Check sheet for the modelled part. Datum: model origin and axes. Units: mm. A direction names the side the tool comes from. Give positions to 0.01 mm unless a question says otherwise; leave off trailing zeros. Order: outer loops, then holes, each group sorted by start corner. A loop starts at its lowest first (then second) coordinate and runs counter-clockwise, first axis right, second up.
Autodesk Inventor part; units mm, degrees
ref_plane "РабПлоскость1" through (-1, 17.5, -4.0985) normal (0, 0, -1) x (-1, 0, 0)
ref_plane "YZ Plane" through (0, 0, 0) normal (1, 0, 0) x (0, 1, 0)
ref_plane "XZ Plane" through (0, 0, 0) normal (0, 1, 0) x (-1, 0, 0)
sketch "Эскиз1" plane through (0, 0, 0) normal (1, 0, 0) x (0, 1, 0)
  line L0 (0, 0) -> (0, -8.197)
  circle A0 centre (0, 0) radius 1.5
  circle A1 centre (0, -8.197) radius 1.5
  line L1 (-2.5, 2.4015) -> (2.5, 2.4015)
  line L2 (2.5, 2.4015) -> (2.5, -10.5985)
  line L3 (2.5, -10.5985) -> (-2.5, -10.5985)
  line L4 (-2.5, -10.5985) -> (-2.5, 2.4015)
  line L5 (-2.5, 2.4015) -> (2.5, -10.5985) construction
  line L6 (2.5, 2.4015) -> (-2.5, -10.5985) construction
  point P0 (0, -4.0985)
  dimension "d0" = 8.197
  dimension "d1" = 3
  dimension "d2" = 3
  dimension "d3" = 5
  dimension "d4" = 13
extrude "Выдавливание1" add sketch "Эскиз1" along normal blind 5
sketch "Эскиз2" plane through (0, 2.5, 2.4015) normal (0, 1, 0) x (1, 0, 0)
  line L0 (0, 0) -> (5, 0)
  line L1 (2.5, 0) -> (2.5, 13)
  line L2 (0, 13) -> (5, 13)
  line L3 (0, 13) -> (0, 0)
  line L4 (5, 4) -> (0, 4)
  line L5 (0, 4) -> (0, 9)
  line L6 (0, 9) -> (5, 9)
  line L7 (5, 9) -> (5, 4)
  line L8 (5, 4) -> (0, 9) construction
  line L9 (0, 4) -> (5, 9) construction
  point P0 (0, 2.4015)
  point P1 (2.5, 6.5)
  dimension "d7" = 5
extrude "Выдавливание2" add sketch "Эскиз2" along normal blind 15 contours L3 L6 L1 L4 | L1 L6 L7 L4
sketch "Эскиз3" plane through (0, 0, 0) normal (-1, 0, 0) x (0, 0, 1)
  line L0 (-1.5985, 17.5) -> (-6.5985, 17.5)
  line L1 (-4.0985, 17.5) -> (-4.0985, 16)
  line L2 (-9.0985, 14.5) -> (0.9015, 14.5)
  line L3 (0.9015, 14.5) -> (0.9015, 17.5)
  line L4 (0.9015, 17.5) -> (-9.0985, 17.5)
  line L5 (-9.0985, 17.5) -> (-9.0985, 14.5)
  line L6 (-9.0985, 14.5) -> (0.9015, 17.5) construction
  line L7 (0.9015, 14.5) -> (-9.0985, 17.5) construction
  point P0 (0, 0)
  dimension "d10" = 1.5
  dimension "d11" = 10
  dimension "d12" = 3
extrude "Выдавливание3" add sketch "Эскиз3" along normal blind 10
sketch "Эскиз4" plane through (0, 17.5, 2.4015) normal (0, 1, 0) x (1, 0, 0)
  line L0 (0, 1.5) -> (-10, 1.5)
  line L1 (-5, 1.5) -> (-5, 11.5)
  line L2 (0, 11.5) -> (-10, 11.5)
  circle A0 centre (-5, 6.5) radius 4
  line L3 (-10, 1.5) -> (-10, 11.5)
  line L4 (-10, 1.5) -> (-10, 11.5)
  point P0 (0, 2.4015)
  point P1 (-7.0808, 9.9162)
  point P2 (-7.0808, 3.0838)
  dimension "d15" = 8
extrude "Выдавливание4" cut sketch "Эскиз4" against normal blind 10 contours A0 L1 | L1 A0
chamfer "Фаска1" distance 2.5 angle 45 2 edges at (0, 16, -1.5985) (0, 16, -6.5985)
chamfer "Фаска2" distance 4 angle 45 2 edges at (2.5, 2.5, -6.5985) (2.5, 2.5, -1.5985)
sketch "Эскиз5" plane through (-10, 0, 0) normal (-1, 0, 0) x (0, 0, 1)
  line L0 (-9.0985, 14.5) -> (0.9015, 14.5)
  line L1 (-9.0985, 14.5) -> (-12.0985, 14.5)
  line L2 (0.9015, 17.5) -> (-9.0985, 17.5)
  line L3 (-12.0985, 14.5) -> (-9.0985, 14.5)
  line L4 (-9.0985, 14.5) -> (-9.0985, 17.5)
  line L5 (-9.0985, 17.5) -> (-12.0985, 17.5)
  line L6 (-12.0985, 17.5) -> (-12.0985, 14.5)
  line L7 (0.9015, 17.5) -> (3.9015, 17.5)
  line L8 (3.9015, 17.5) -> (3.9015, 14.5)
  line L9 (3.9015, 14.5) -> (0.9015, 14.5)
  line L10 (0.9015, 14.5) -> (0.9015, 17.5)
  line L11 (-9.0985, 17.5) -> (0.9015, 17.5)
  line L12 (0.9015, 17.5) -> (0.9015, 14.5)
  line L13 (0.9015, 14.5) -> (-9.0985, 14.5)
  line L14 (-9.0985, 14.5) -> (-9.0985, 17.5)
  point P0 (0, 0)
  dimension "d24" = 3
  dimension "d25" = 3
  dimension "d26" = 3
extrude "Выдавливание5" cut sketch "Эскиз5" against normal blind 4
sketch "Эскиз6" plane through (-6, 0, 0) normal (-1, 0, 0) x (0, 0, 1)
  line L0 (-9.0985, 17.5) -> (-9.0985, 14.5)
  line L1 (-9.0985, 17.5) -> (-12.0985, 17.5)
  line L2 (-12.0985, 17.5) -> (-12.0985, 14.5)
  line L3 (-12.0985, 14.5) -> (-9.0985, 14.5)
  line L4 (-9.0985, 14.5) -> (-9.0985, 17.5)
  line L5 (-1.5985, 14.5) -> (-6.5985, 14.5)
  line L6 (-4.0985, 14.5) -> (-4.0985, 15.1912)
  line L7 (-12.0985, 17.5) -> (-10.5985, 17.5)
  line L8 (-12.0985, 16) -> (-12.0985, 17.5)
  circle A0 centre (-10.5985, 16) radius 0.75
  point P0 (0, 0)
  dimension "d29" = 3
  dimension "d30" = 3
  dimension "d33" = 1.5
ref_plane "РабПлоскость1" through (-1, 17.5, -4.0985) normal (0, 0, -1) x (-1, 0, 0)
extrude "Выдавливание6" add sketch "Эскиз6" against normal blind 4
mirror "Зеркальное отражение1" about plane through (-1, 17.5, -4.0985) normal (0, 0, -1) of "Выдавливание6"
sketch "Эскиз7" plane through (-6, 0, 0) normal (-1, 0, 0) x (0, 0, 1)
  line L0 (-7.9715, 17.5) -> (-12.0985, 17.5)
  circle A0 centre (-10.5985, 16) radius 0.75
  line L1 (-7.9715, 14.5) -> (-12.0985, 14.5)
  line L2 (-7.9715, 17.5) -> (-7.9715, 14.5)
  line L3 (-7.9715, 17.5) -> (-12.0985, 17.5)
  line L4 (-12.0985, 17.5) -> (-12.0985, 14.5)
  circle A1 centre (2.4015, 16) radius 0.75
  line L5 (-0.2255, 14.5) -> (-0.2255, 17.5)
  line L6 (3.9015, 14.5) -> (-0.2255, 14.5)
  line L7 (3.9015, 17.5) -> (3.9015, 14.5)
  line L8 (-0.2255, 17.5) -> (3.9015, 17.5)
  line L9 (-7.9715, 17.5) -> (-7.9715, 14.5)
  line L10 (-0.2255, 14.5) -> (-7.9715, 14.5)
  line L11 (-0.2255, 14.5) -> (-0.2255, 17.5)
  line L12 (-7.9715, 17.5) -> (-0.2255, 17.5)
  point P0 (0, 0)
chamfer "Фаска3" distance 2.5 angle 45 3 edges at (2.4995, 16, -1.5985) (2.4995, 16, -6.5985) (5, 17.5, -4.0985)
properties part number "КВ33.044.207 - Крепление вакумной присоски"
1) Section check A-A, the plane x = -5. Record the cut outline in (y, z).
Recorded:
outline: (14.5, -12.1) - (17.5, -12.1) - (17.5, -8.1) - (14.5, -8.1) - close; (14.5, -0.1) - (17.5, -0.1) - (17.5, 3.9) - (14.5, 3.9) - close; hole circle Ø1.5 at (16, -10.6); hole circle Ø1.5 at (16, 2.4)
2) Section check B-B, the plane y = 0. Record the cut outline in (x, z), then the cut area to 3 significant figures.
Recorded:
outline: (0, -10.6) - (5, -10.6) - (5, -9.7) - (0, -9.7) - close; (0, -6.7) - (5, -6.7) - (5, -1.5) - (0, -1.5) - close; (0, 1.5) - (5, 1.5) - (5, 2.4) - (0, 2.4) - close
area: 35.0 mm2
3) Section check D-D, the plane x = 1.25. State how many separate pieces and enclosed holes the cut face has, then the cut area to 3 significant figures.
Recorded:
separate pieces: 1
enclosed holes: 2
area: 151 mm2
4) Depth check by flat-ended pin: pin 1 Ø1.5 at (y, z) = (15.5, -10.5) entering from +X; pin 2 Ø4 at (x, y) = (3, 0) entering from -Z; pin 3 Ø1.5 at (x, y) = (2, 1) entering from +Z; pin 4 Ø1.5 at (x, y) = (-1.5, 14.5) entering from +Z. Enter the tip coordinate at first touch or a pass-through.
Recorded:
pin 1: stops at x = -2
pin 2: stops at z = -10.6
pin 3: stops at z = 2.4
pin 4: stops at z = 3.9
5) Set-up check for faces 4 (the face through (2.5, 4.5, 0.4)), 5 (the face through (2, 11, -6.598)), 6 (the face through (-1, 16, 0.902)), 7 (the face through (0, 4, -4)): record each of +Z, -Z, +X, -X, +Y, -Y from which the full face is reachable in a straight line by a thin tool's end or side.
Recorded:
face 4: +Z, +X, -X
face 5: -Z, +X, -X
face 6: +Z, +X, +Y, -Y
face 7: +Z, -Z, -X, -Y
6) Draft check along Y on faces 1 (the face through (2, 0, 2.402)), 2 (the face through (0, 17.5, -4)), 3 (the face through (3, 11, -1.598)). Enter one of: +Y half, -Y half, draft (parallel to the pull), parting line (faces both ways), or undercut.
Recorded:
face 1: draft
face 2: +Y half
face 3: undercut
7) Material ranges on L1, parallel to Z at x = 3.15, y = 0; L2, parallel to Z at x = 4, y = -0.75; L3, parallel to Z at x = 0.25, y = 10.5, recorded low to high.
Recorded:
L1: z = -10.6 to -9.7, -6.7 to -1.5, 1.5 to 2.4
L2: z = -10.6 to -9.5, -6.9 to -1.3, 1.3 to 2.4
L3: z = -6.6 to -1.6
